from build123d import *

# Parameters (mm, degrees)
SKETCH_1_W            = 34
SKETCH_1_H            = 40
SKETCH_1_R            = 9.5
SKETCH_1_R_2          = 1.5
EXTRUDE_1_DEPTH       = 2
HOLE_WIZARD_3_0_3_1_D = 3
FILLET_1_R            = 2
SKETCH_5_W            = 10
SKETCH_5_H            = 2
EXTRUDE_2_DEPTH       = 5
FILLET_2_R            = 2
CHAMFER_1_SIZE        = 1.5


with BuildPart() as part:
    # 草图1 → 凸台-拉伸1 (new body)
    with BuildSketch(Plane(origin=(0, 0, 0), x_dir=(1, 0, 0), z_dir=(0, 1, 0))):
        with Locations((17, 20)):
            Rectangle(SKETCH_1_W, SKETCH_1_H)
        with Locations(Location((17, 20, 0), (0, 0, 270))):
            Circle(SKETCH_1_R, mode=Mode.SUBTRACT)
        with Locations(Location((26.192388155, 29.192388155, 0), (0, 0, 270))):
            Circle(SKETCH_1_R_2, mode=Mode.SUBTRACT)
        with Locations(Location((7.807611845, 29.192388155, 0), (0, 0, 270))):
            Circle(SKETCH_1_R_2, mode=Mode.SUBTRACT)
        with Locations(Location((7.807611845, 10.807611845, 0), (0, 0, 270))):
            Circle(SKETCH_1_R_2, mode=Mode.SUBTRACT)
        with Locations(Location((26.192388155, 10.807611845, 0), (0, 0, 270))):
            Circle(SKETCH_1_R_2, mode=Mode.SUBTRACT)
    extrude(amount=EXTRUDE_1_DEPTH)

    # Ø3.0 (3) 直径孔1 (through all)
    with Locations(Plane(origin=(3, 2, -37), x_dir=(0, 0, 1), z_dir=(0, 1, 0))):
        with Locations((0, 0), (0, 28), (34, 28), (34, 0)):
            Hole(HOLE_WIZARD_3_0_3_1_D / 2)

    # 圆角1
    fillet_1_edges = [part.edges().sort_by_distance(p)[0] for p in [
        (0, 1, -40),
        (34, 1, -40),
        (34, 1, 0),
        (0, 1, 0),
    ]]
    fillet(fillet_1_edges, radius=FILLET_1_R)

    # 草图5 → 凸台-拉伸2 (add)
    with BuildSketch(Plane.XZ):
        with Locations((17, 1)):
            Rectangle(SKETCH_5_W, SKETCH_5_H)
        with Locations((17, -41)):
            Rectangle(SKETCH_5_W, SKETCH_5_H)
    extrude(amount=-EXTRUDE_2_DEPTH)

    # 圆角2
    fillet_2_edges = [part.edges().sort_by_distance(p)[0] for p in [
        (22, 1, -40),
        (12, 1, -40),
        (12, 1, 0),
        (22, 1, 0),
    ]]
    fillet(fillet_2_edges, radius=FILLET_2_R - 0.0001)  # a hair under: the kernel refuses the full size

    # 倒角1
    chamfer_1_edges = [part.edges().sort_by_distance(p)[0] for p in [
        (26.192388155, 2, -30.692388155),
        (7.807611845, 2, -30.692388155),
        (7.807611845, 2, -12.307611845),
        (26.192388155, 2, -12.307611845),
    ]]
    chamfer(chamfer_1_edges, length=CHAMFER_1_SIZE)


solid = part.part
Here's how the part is built. I have some questions about the finished solid (model axes, mm). A direction names the side the tool comes from. Round coordinates to 2 decimals unless told otherwise and drop trailing zeros. Order: outer loops, then holes, each group sorted by start corner. A loop starts at its lowest first (then second) coordinate and runs counter-clockwise, first axis right, second up. Notation, with made-up numbers: (48, -22) -> (101, -22) arc R17 ccw to (101, 7) -> close; hole circle Ø2 at (57, 13). An arc over 180 degrees is marked (long way). Return JSON: item names as keys, results as strings.
Q1. If we section it at D-D on x = 17: List the corners of the cut face in (y, z) for me, plus the area to 3 significant figures.
Filled sheet:
{"outline": "(0, -42) -> (5, -42) -> (5, -40) -> (2, -40) -> (2, -29.5) -> (0, -29.5) -> close; (0, -10.5) -> (2, -10.5) -> (2, 0) -> (5, 0) -> (5, 2) -> (0, 2) -> close", "area": "62.0 mm^2"}
Q2. I need wall thicknesses on line 1 along X through (y, z) = (0.75, -3); line 2 along Z through (x, y) = (18.5, 3.05); line 3 along Y through (x, z) = (32, -15.5). Which ranges of each line are inside material? Lowest first, please. Write a range as from..to.
Filled sheet:
{"line 1": "x = 0..1.5, 4.5..29.5, 32.5..34", "line 2": "z = -42..-40, 0..2", "line 3": "y = 0..2"}
Q3. If we section it at B-B on z = -20: List the corners of the cut face in (x, y) for me, plus the area to 3 significant figures.
Filled sheet:
{"outline": "(0, 0) -> (7.5, 0) -> (7.5, 2) -> (0, 2) -> close; (26.5, 0) -> (34, 0) -> (34, 2) -> (26.5, 2) -> close", "area": "30.0 mm^2"}
Q4. If we section it at C-C on z = -37: List the corners of the cut face in (x, y) for me, plus the area to 3 significant figures.
Filled sheet:
{"outline": "(0, 0) -> (1.5, 0) -> (1.5, 2) -> (0, 2) -> close; (4.5, 0) -> (29.5, 0) -> (29.5, 2) -> (4.5, 2) -> close; (32.5, 0) -> (34, 0) -> (34, 2) -> (32.5, 2) -> close", "area": "56.0 mm^2"}
Q5. If we section it at A-A on x = 3: List the corners of the cut face in (y, z) for me, plus the area to 3 significant figures.
Filled sheet:
{"outline": "(0, -40) -> (2, -40) -> (2, -38.5) -> (0, -38.5) -> close; (0, -35.5) -> (2, -35.5) -> (2, -4.5) -> (0, -4.5) -> close; (0, -1.5) -> (2, -1.5) -> (2, 0) -> (0, 0) -> close", "area": "68.0 mm^2"}
Q6. For pin 1 Ø1.6 at (y, z) = (1.5, 1) entering from -X; pin 2 Ø5 at (x, z) = (26.19, -29.19) entering from -Y; pin 3 Ø3 at (x, z) = (4, -28.5) entering from +Y; pin 4 Ø0.6 at (x, y) = (7.5, 0.5) entering from -Z, each with a flat end and sliding along its axis, tell me the tip position at first contact or that it passes through.
Filled sheet:
{"pin 1": "stops at x = 10.87", "pin 2": "stops at y = 0", "pin 3": "stops at y = 2", "pin 4": "stops at z = -40"}
Q7. If we mould it in two halves opening along Z, with no side actions, what happens to faces 1 (the flat face through (17, 3, -40)), 2 (the cylindrical face through (22.57, 1.01, 0.6)), 3 (the cylindrical face through (0.57, 1.01, -39.4)), 4 (the flat face through (22, 4, -41))? For each: released by +Z, released by -Z, zero draft, split by the parting line, or undercut.
Filled sheet:
{"face 1": "undercut", "face 2": "released by +Z", "face 3": "released by -Z", "face 4": "zero draft"}
Q8. Which directions (+Z, -Z, +X, -X, +Y, -Y) give clear straight access to the entire face, cutting with the end or side of a thin tool? Please do faces 5 (the flat face through (34, 1, -20)), 6 (the flat face through (17, 3, 0)).
Filled sheet:
{"face 5": "+Z, -Z, +X, +Y, -Y", "face 6": "+X, -X, +Y"}
